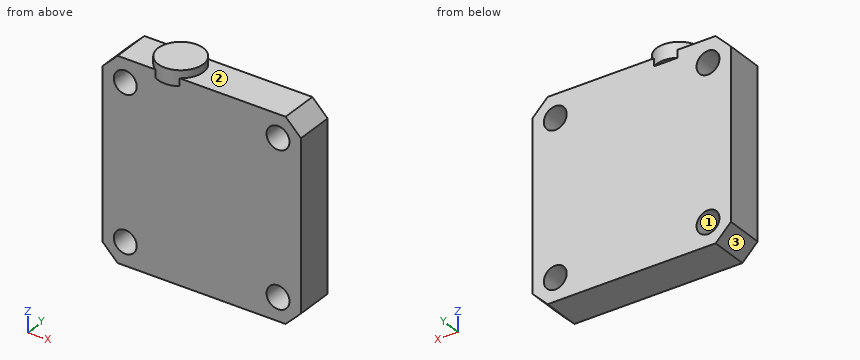
from build123d import *

# Parameters (mm, degrees)
SKETCH1_R           = 1.5
BOSS_EXTRUDE1_DEPTH = 5
SKETCH2_R           = 2.950338073
BOSS_EXTRUDE2_DEPTH = 1


with BuildPart() as part:
    # Sketch1 → Boss-Extrude1 (new body)
    with BuildSketch(Plane(origin=(0, 0, 0), x_dir=(1, 0, 0), z_dir=(0, 1, 0))):
        Polygon((-11, 13), (-13, 11), (-13, -11), (-11, -13), (11, -13), (13, -11), (13, 11), (11, 13), align=None)
        with Locations(Location((-10, 10, 0), (0, 0, 270))):
            Circle(SKETCH1_R, mode=Mode.SUBTRACT)
        with Locations(Location((10, 10, 0), (0, 0, 270))):
            Circle(SKETCH1_R, mode=Mode.SUBTRACT)
        with Locations(Location((10, -10, 0), (0, 0, 270))):
            Circle(SKETCH1_R, mode=Mode.SUBTRACT)
        with Locations(Location((-10, -10, 0), (0, 0, 270))):
            Circle(SKETCH1_R, mode=Mode.SUBTRACT)
    extrude(amount=BOSS_EXTRUDE1_DEPTH)

    # Sketch2 → Boss-Extrude2 (add, symmetric)
    with BuildSketch(Plane.XY.offset(13)):
        with Locations(Location((-4.476260218, 2.486184382, 0), (0, 0, 237.423977883))):
            Circle(SKETCH2_R)
    extrude(amount=BOSS_EXTRUDE2_DEPTH, both=True)


solid = part.part
Work out the finished part from the listing and answer in its coordinate system (mm). Face numbers are marked on the shaded views. Give positions to 0.01 mm unless a question says otherwise; leave off trailing zeros. Order: outer loops, then holes, each group sorted by start corner. A loop starts at its lowest first (then second) coordinate and runs counter-clockwise, first axis right, second up. Notation, with made-up numbers: (72, 79) -> (106, 79) arc R13 cw to (106, 91) -> close; hole circle Ø10 at (-20, -39.75). An arc over 180 degrees is marked (long way). One line per item, written item: value.
Item 1: Find section D-D, the plane z = 1.25. Give the vertices of the cut face in (x, y), plus the area to 3 significant figures.
Answer sheet:
outline: (-13, 0) -> (13, 0) -> (13, 5) -> (-13, 5) -> close
area: 130 mm²
Item 2: Find section B-B, the plane x = -10. Give the vertices of the cut face in (y, z), plus the area to 3 significant figures.
Answer sheet:
outline: (0, -13) -> (5, -13) -> (5, -11.5) -> (0, -11.5) -> close; (0, -8.5) -> (5, -8.5) -> (5, 8.5) -> (0, 8.5) -> close; (0, 11.5) -> (5, 11.5) -> (5, 13) -> (0, 13) -> close
area: 100 mm²
Item 3: Find section C-C, the plane y = 2.6. Give the vertices of the cut face in (x, z).
Answer sheet:
outline: (-13, -11) -> (-11, -13) -> (11, -13) -> (13, -11) -> (13, 11) -> (11, 13) -> (-1.53, 13) -> (-1.53, 14) -> (-7.42, 14) -> (-7.42, 13) -> (-11, 13) -> (-13, 11) -> close; hole circle Ø3 at (-10, -10); hole circle Ø3 at (-10, 10); hole circle Ø3 at (10, -10); hole circle Ø3 at (10, 10)
Item 4: Straight lines are drawn through the part: probe 1 along X at (y, z) = (3.65, -10); probe 2 along X at (y, z) = (3.2, -11); probe 3 along Y at (x, z) = (2.25, 12.75). For each, find the intervals that lie inside material, in ascending order.
Answer sheet:
probe 1: -13 to -11.5, -8.5 to 8.5, 11.5 to 13
probe 2: -13 to -11.12, -8.88 to 8.88, 11.12 to 13
probe 3: 0 to 5
Item 5: Determine the mould class of the marked faces 1, 2 and 3 for opening direction Z: released by +Z, released by -Z, zero draft, split by the parting line, or undercut.
Answer sheet:
face 1: undercut
face 2: released by +Z
face 3: released by -Z
Item 6: Find section A-A, the plane z = -10. Give the vertices of the cut face in (x, y), plus the area to 3 significant figures.
Answer sheet:
outline: (-13, 0) -> (-11.5, 0) -> (-11.5, 5) -> (-13, 5) -> close; (-8.5, 0) -> (8.5, 0) -> (8.5, 5) -> (-8.5, 5) -> close; (11.5, 0) -> (13, 0) -> (13, 5) -> (11.5, 5) -> close
area: 100 mm²
Item 7: Flat-ended cylindrical pins translate along their axes: P1, Ø5, axis at x = 10, z = 10, coming from the +Y side; P2, Ø3.5, axis at x = 10, z = -10, coming from the -Y side; P3, Ø1, axis at x = 7.5, y = 4, coming from the +Z side; P4, Ø2.5, axis at x = -10, z = -10, coming from the +Y side. Find the tip coordinate at first contact, or state that the pin passes through.
Answer sheet:
P1: y = 5
P2: y = 0
P3: z = 13
P4: through
